Here's how the part is built. I have some questions about the finished solid (model axes, mm). Round coordinates to 2 decimals unless told otherwise and drop trailing zeros. Order: outer loops, then holes, each group sorted by start corner. A loop starts at its lowest first (then second) coordinate and runs counter-clockwise, first axis right, second up. Notation, with made-up numbers: (7, 54.5) - (29, 54.5) arc R11 ccw to (29, 66.5) - close; hole circle Ø8 at (-3.5, 78.5). An arc over 180 degrees is marked (long way). Answer as a JSON object with one key per item and string values.
```python
from build123d import *

# Parameters (mm, degrees)
BOSS_EXTRU_1_DEPTH                                 = 15
FRAISAGE_POUR_VIS_T_TE_FRAIS_E_CRUCIFO_D           = 3.2
FRAISAGE_POUR_VIS_T_TE_FRAIS_E_CRUCIFO_CSINK_D     = 6
FRAISAGE_POUR_VIS_T_TE_FRAIS_E_CRUCIFO_CSINK_ANGLE = 92
CONG_2_R                                           = 5


with BuildPart() as part:
    # Esquisse1 → Boss.-Extru.1 (new body)
    with BuildSketch(Plane.XY):
        Polygon((27.5, 6), (-27.5, 6), (-27.5, 1), (-15, 1), (-15, -6), (15, -6), (15, 1), (27.5, 1), align=None)
    extrude(amount=BOSS_EXTRU_1_DEPTH)

    # Fraisage pour vis à tête fraisée cruciforme M31 (through all)
    with Locations(Plane(origin=(0, 6, 0), x_dir=(1, 0, 0), z_dir=(0, 1, 0))):
        with Locations((-20, -7.5), (20, -7.5)):
            CounterSinkHole(FRAISAGE_POUR_VIS_T_TE_FRAIS_E_CRUCIFO_D / 2, FRAISAGE_POUR_VIS_T_TE_FRAIS_E_CRUCIFO_CSINK_D / 2, counter_sink_angle=FRAISAGE_POUR_VIS_T_TE_FRAIS_E_CRUCIFO_CSINK_ANGLE)

    # Congé2
    cong_2_edges = [part.edges().sort_by_distance(p)[0] for p in [
        (-15, -2.5, 15),
        (-27.5, 3.5, 0),
        (0, -6, 15),
        (15, -6, 7.5),
        (-15, -6, 7.5),
        (15, -2.5, 15),
        (27.5, 3.5, 15),
        (-27.5, 3.5, 15),
        (27.5, 3.5, 0),
        (15, -2.5, 0),
        (0, -6, 0),
        (-15, -2.5, 0),
    ]]
    fillet(cong_2_edges, radius=CONG_2_R)


solid = part.part
```
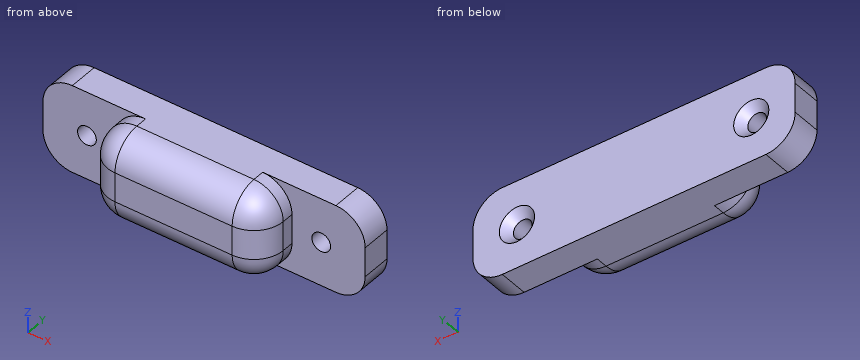
1. For P1, Ø1, axis at y = 0, z = 6.5, coming from the +X side; P2, Ø1, axis at x = 2, z = 4.5, coming from the -Y side; P3, Ø2, axis at x = 21, z = 8.5, coming from the -Y side; P4, Ø1.9, axis at x = -20, z = 7.5, coming from the -Y side, each with a flat end and sliding along its axis, tell me the tip position at first contact or that it passes through.
Responses:
{"P1": "x = 15", "P2": "y = -6", "P3": "y = 1", "P4": "through"}
2. Imagine slicing it at A-A (z = 7.5). List the corners of the cut face in (x, y) for me, plus the area to 3 significant figures.
Responses:
{"outline": "(-27.5, 1) - (-21.6, 1) - (-21.6, 4.65) - (-23, 6) - (-27.5, 6) - close; (-18.4, 1) - (-15, 1) - (-15, -1) arc R5 ccw to (-10, -6) - (10, -6) arc R5 ccw to (15, -1) - (15, 1) - (18.4, 1) - (18.4, 4.65) - (17, 6) - (-17, 6) - (-18.4, 4.65) - close; (21.6, 1) - (27.5, 1) - (27.5, 6) - (23, 6) - (21.6, 4.65) - close", "area": "438 mm2"}
3. Imagine slicing it at B-B (y = 2.75). List the corners of the cut face in (x, z) for me.
Responses:
{"outline": "(-27.5, 5) arc R5 ccw to (-22.5, 0) - (22.5, 0) arc R5 ccw to (27.5, 5) - (27.5, 10) arc R5 ccw to (22.5, 15) - (-22.5, 15) arc R5 ccw to (-27.5, 10) - close; hole circle Ø3.2 at (-20, 7.5); hole circle Ø3.2 at (20, 7.5)"}
4. Imagine slicing it at C-C (x = 20). List the corners of the cut face in (y, z) for me, plus the area to 3 significant figures.
Responses:
{"outline": "(1, 0) - (6, 0) - (6, 4.5) - (4.65, 5.9) - (1, 5.9) - close; (1, 9.1) - (4.65, 9.1) - (6, 10.5) - (6, 15) - (1, 15) - close", "area": "57.1 mm2"}
5. If I drill on L1, parallel to X at y = 2.15, z = 7.5; L2, parallel to Z at x = 20, y = 3.4; L3, parallel to Y at x = 15, z = 13.5, over which ranges is the centre line in solid material (lowest first)? Write a range as [from, to].
Responses:
{"L1": "[-27.5, -21.6], [-18.4, 18.4], [21.6, 27.5]", "L2": "[0, 5.9], [9.1, 15]", "L3": "[1, 6]"}
6. Imagine slicing it at D-D (x = -13). List the corners of the cut face in (y, z) for me.
Responses:
{"outline": "(-5, 5) arc R4 ccw to (-1, 1) - (1, 1) - (1, 0) - (6, 0) - (6, 15) - (1, 15) - (1, 14) - (-1, 14) arc R4 ccw to (-5, 10) - close"}
